Read the model definition and answer for the solid it produces. Units are mm, in the model's axes. Face numbers are marked on the shaded views. A direction names the side the tool comes from. Round coordinates to 2 decimals unless told otherwise and drop trailing zeros. Order: outer loops, then holes, each group sorted by start corner. A loop starts at its lowest first (then second) coordinate and runs counter-clockwise, first axis right, second up. Notation, with made-up numbers: (-30, 7) - (-5, 7) arc R14 ccw to (-5, 24) - close; hole circle Ø5 at (-13, 77.5). An arc over 180 degrees is marked (long way). One line per question, with ' | ' between items. Start each with the question number.
1) For the marked faces 4 and 5, determine the directions among +Z, -Z, +X, -X, +Y, -Y from which every point of the face is accessible in a straight line to the end or side of a thin tool.
2) The part is cut by section C-C, the plane z = 5.5. Give the vertices of the cut face in (x, y).
3) The mould has two halves that part along Y. Classify the marked faces 1, 2 and 3: pulls with the +Y half, pulls with the -Y half, needs draft (parallel to the pull), parting line crosses it, or undercut.
4) Flat-ended cylindrical pins translate along their axes: pin 1 (1 mm diameter, centred on x = -32.5, z = 5, fed in from +Y); pin 2 (4 mm diameter, centred on x = 22.5, z = 2, fed in from -Y); pin 3 (2 mm diameter, centred on x = 40, z = 3.5, fed in from +Y). Find the tip coordinate at first contact, or state that the pin passes through.
5) The part is cut by section D-D, the plane z = 11.5. Give the vertices of the cut face in (x, y), plus the area to 3 significant figures.
6) Straight lines are drawn through the part: line 1 (Y direction, x = 0, z = 2.75); line 2 (Y direction, x = -7, z = 1); line 3 (X direction, y = 10, z = 2). For each, find the intervals that lie inside material, in ascending order. Write a range as from..to.
7) The part is cut by section A-A, the plane x = 0. Give the vertices of the cut face in (y, z).
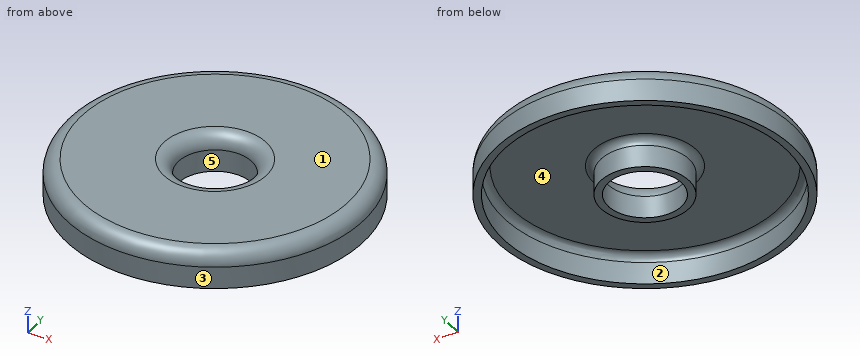
from build123d import *

# Parameters (mm, degrees)
F0_R     = 51.33938
F0_R_2   = 12.7
F1_DEPTH = 12.7
F2_R     = 5.08
F3_T     = -2.54


with BuildPart() as f1:
    # F0 (on Top) → F1 (new body)
    with BuildSketch(Plane.XY):
        Circle(F0_R)
        Circle(F0_R_2, mode=Mode.SUBTRACT)
    extrude(amount=F1_DEPTH)

    # F2
    f2_edges = [f1.edges().sort_by_distance(p)[0] for p in [
        (-51.33938, 0, 12.7),
        (-12.7, 0, 12.7),
    ]]
    fillet(f2_edges, radius=F2_R)

    # F3
    f3_openings = [f1.faces().sort_by_distance(p)[0] for p in [
        (-49.887283, 0, 0),
    ]]
    offset(amount=F3_T, openings=f3_openings)


solid = f1.part
Values:
1) face 4: -Z | face 5: +Z, -Z
2) outline: circle Ø102.68 at (0, 0); circle Ø30.48 at (0, 0); hole circle Ø97.6 at (0, 0); hole circle Ø25.4 at (0, 0)
3) face 1: needs draft | face 2: undercut | face 3: parting line crosses it
4) pin 1: stops at y = 40.15 | pin 2: stops at y = -47.07 | pin 3: stops at y = 33.39
5) outline: circle Ø99.08 at (0, 0); hole circle Ø29 at (0, 0) | area: 7,050 mm^2
6) line 1: y = -51.34..-48.8, -15.24..-12.7, 12.7..15.24, 48.8..51.34 | line 2: y = -50.86..-48.29, -13.54..-10.6, 10.6..13.54, 48.29..50.86 | line 3: x = -50.36..-47.76, -11.5..-7.83, 7.83..11.5, 47.76..50.36
7) outline: (-51.34, 0) - (-48.8, 0) - (-48.8, 7.62) arc R2.54 cw to (-46.26, 10.16) - (-17.78, 10.16) arc R2.54 cw to (-15.24, 7.62) - (-15.24, 0) - (-12.7, 0) - (-12.7, 7.62) arc R5.08 ccw to (-17.78, 12.7) - (-46.26, 12.7) arc R5.08 ccw to (-51.34, 7.62) - close; (12.7, 0) - (15.24, 0) - (15.24, 7.62) arc R2.54 cw to (17.78, 10.16) - (46.26, 10.16) arc R2.54 cw to (48.8, 7.62) - (48.8, 0) - (51.34, 0) - (51.34, 7.62) arc R5.08 ccw to (46.26, 12.7) - (17.78, 12.7) arc R5.08 ccw to (12.7, 7.62) - close
